Part print with two shaded views. Sizes in mm from the minimum x, y, z corner. Give positions to 0.01 mm unless a question says otherwise; leave off trailing zeros. Loops run counter-clockwise (first coordinate to the right, second up) from the corner with the lowest first, then second, coordinate; pieces in that order, holes last. Notation, with made-up numbers: M -20,76 L -1,76 A26 ccw -1,103 Z; hole C 89.5,37.5 d11. An arc over 180 degrees is marked long. Answer in a Markdown table with one row per item.
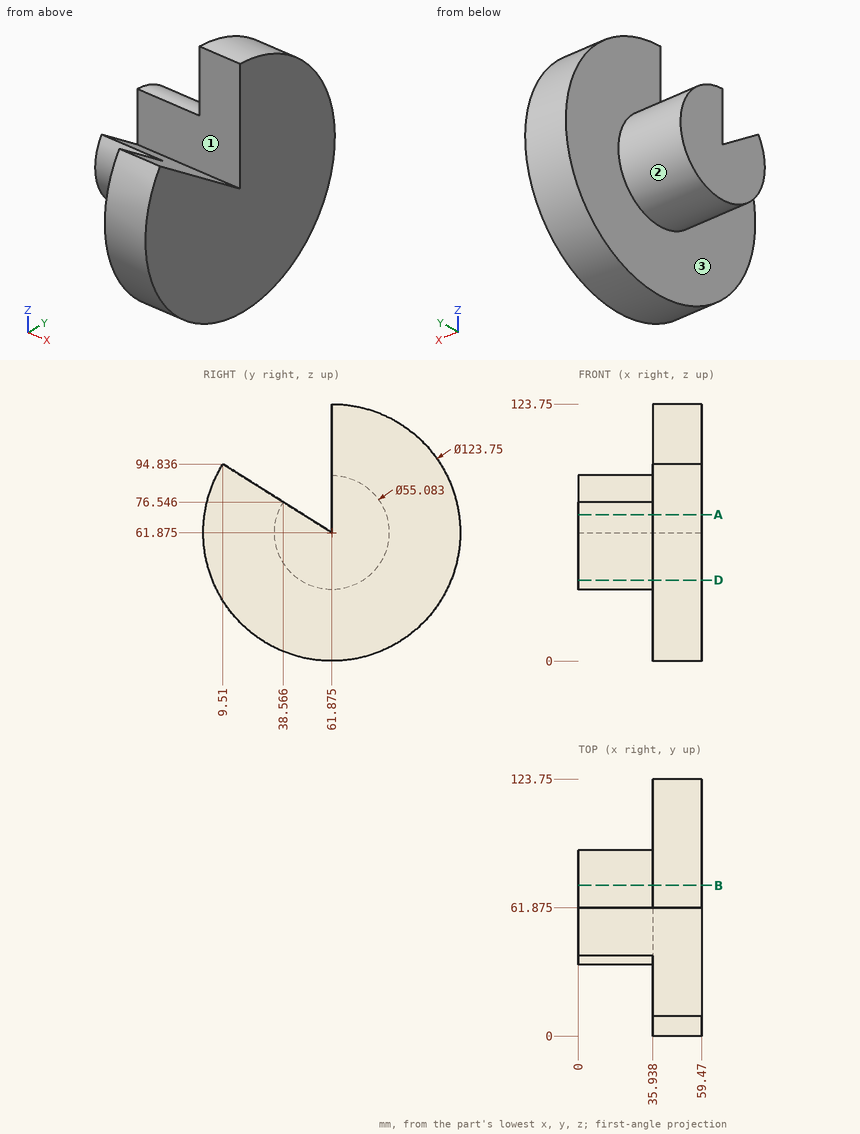
Q1. Probe probe 1 along X at (y, z) = (90.5, 36.5); probe 2 along Z at (x, y) = (42, 63.5); probe 3 along Y at (x, z) = (12, 73) (1 decimal). List the from-to ranges inside material, lowest first.
Reported:
| item | result |
|---|---|
| probe 1 | 35.94 to 59.47 |
| probe 2 | 0.02 to 123.73 |
| probe 3 | 36.7 to 44.2, 61.9 to 87.1 |
Q2. Saw through at B-B (y = 72.5). Give the cut face in (x, z) (1 decimal).
Reported:
| item | result |
|---|---|
| outline | M 0,36.5 L 35.9,36.5 L 35.9,0.9 L 59.5,0.9 L 59.5,122.8 L 35.9,122.8 L 35.9,87.3 L 0,87.3 Z |
Q3. Saw through at A-A (z = 70.5). Give the cut face in (x, y) (1 decimal).
Reported:
| item | result |
|---|---|
| outline | M 0,35.7 L 35.9,35.7 L 35.9,0.6 L 59.5,0.6 L 59.5,48.2 L 0,48.2 Z; M 0,61.9 L 59.5,61.9 L 59.5,123.1 L 35.9,123.1 L 35.9,88 L 0,88 Z |
Q4. Saw through at D-D (z = 39). Give the cut face in (x, y).
Reported:
| item | result |
|---|---|
| outline | M 0,46.54 L 35.94,46.54 L 35.94,4.38 L 59.47,4.38 L 59.47,119.37 L 35.94,119.37 L 35.94,77.21 L 0,77.21 Z |
Q5. Mould opens along Y. For the marked faces 1, 2 and 3 say: released by +Y, released by -Y, zero draft, split by the parting line, or undercut.
Reported:
| item | result |
|---|---|
| face 1 | undercut |
| face 2 | split by the parting line |
| face 3 | zero draft |
Q6. Drop flat-ended pins along their axis: pin 1 (4 mm diameter, centred on x = 44.5, y = 29.5, fed in from -Z); pin 2 (5 mm diameter, centred on x = 7, y = 55, fed in from -Z); pin 3 (4 mm diameter, centred on x = 44.5, z = 57, fed in from +Y). Give the stop position or say it passes through.
Reported:
| item | result |
|---|---|
| pin 1 | z = 7.97 |
| pin 2 | z = 34.68 |
| pin 3 | y = 123.68 |
